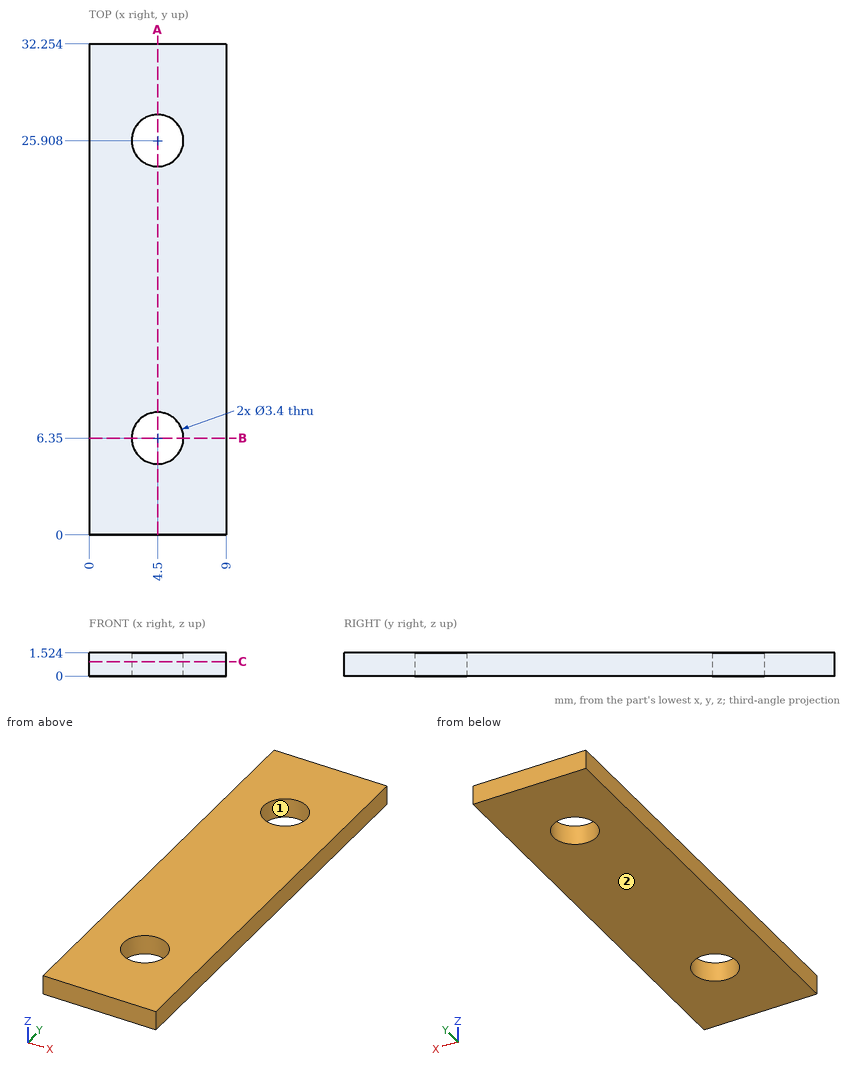
Source: three-view drawing plus pictorial views. Frame: mm from the lowest corner of the part. Round coordinates to 2 decimals unless told otherwise and drop trailing zeros. Loops run counter-clockwise (first coordinate to the right, second up) from the corner with the lowest first, then second, coordinate; pieces in that order, holes last.
Q1. Material intervals for L1, parallel to Y at x = 4.5, z = 1.2; L2, parallel to Y at x = 5.5, z = 1.1 (1 decimal); L3, parallel to X at y = 5, z = 0.5, sorted ascending.
Q2. Section C-C on z = 0.95. Return loops of the section in (x, y), plus the area to 3 significant figures.
Q3. Section B-B on y = 6.35. Return loops of the section in (x, z).
Q4. Pin query (flat end, axial travel): P1, Ø3, axis at x = 3.5, y = 26, coming from the +Z side. Return the tip coordinate at first contact, or that it passes through.
Q5. Pull-direction query (X, two-part tool) for the marked faces 1 and 2; classes: released by +X, released by -X, zero draft, split by the parting line, or undercut.
Q6. Section A-A on x = 4.5. Return loops of the section in (y, z).
Evaluation:
1. L1: y = 0 to 4.65, 8.05 to 24.21, 27.61 to 32.25
1. L2: y = 0 to 5, 7.7 to 24.5, 27.3 to 32.3
1. L3: x = 0 to 3.47, 5.53 to 9
2. outline: (0, 0) - (9, 0) - (9, 32.25) - (0, 32.25) - close; hole circle Ø3.4 at (4.5, 6.35); hole circle Ø3.4 at (4.5, 25.91)
2. area: 272 mm2
3. outline: (0, 0) - (2.8, 0) - (2.8, 1.52) - (0, 1.52) - close; (6.2, 0) - (9, 0) - (9, 1.52) - (6.2, 1.52) - close
4. P1: stops at z = 1.52
5. face 1: undercut
5. face 2: zero draft
6. outline: (0, 0) - (4.65, 0) - (4.65, 1.52) - (0, 1.52) - close; (8.05, 0) - (24.21, 0) - (24.21, 1.52) - (8.05, 1.52) - close; (27.61, 0) - (32.25, 0) - (32.25, 1.52) - (27.61, 1.52) - close
